from build123d import *

# Parameters (mm, degrees)
SKETCH2_W           = 38.1
SKETCH2_H           = 63.5
SKETCH2_R           = 2.1844
SKETCH2_W_2         = 19.939
SKETCH2_H_2         = 40.005
BOSS_EXTRUDE1_DEPTH = 3.175
SKETCH4_W           = 71.079825169
SKETCH4_H           = 63.5
SKETCH4_R           = 14.2875
SKETCH4_R_2         = 2.54
BOSS_EXTRUDE3_DEPTH = 3.175


with BuildPart() as part:
    # Sketch2 → Boss-Extrude1 (new body)
    with BuildSketch(Plane(origin=(0, 0, 0), x_dir=(1, 0, 0), z_dir=(0, 1, 0))):
        with Locations((0, -10.3505)):
            Rectangle(SKETCH2_W, SKETCH2_H)
        with Locations(Location((5.08, 13.462, 0), (0, 0, 270))):
            Circle(SKETCH2_R, mode=Mode.SUBTRACT)
        with Locations(Location((-5.08, 13.462, 0), (0, 0, 270))):
            Circle(SKETCH2_R, mode=Mode.SUBTRACT)
        with Locations(Location((-5.08, -34.163, 0), (0, 0, 270))):
            Circle(SKETCH2_R, mode=Mode.SUBTRACT)
        with Locations(Location((5.08, -34.163, 0), (0, 0, 270))):
            Circle(SKETCH2_R, mode=Mode.SUBTRACT)
        with Locations((0, -10.3505)):
            Rectangle(SKETCH2_W_2, SKETCH2_H_2, mode=Mode.SUBTRACT)
    extrude(amount=BOSS_EXTRUDE1_DEPTH)

    # Sketch4 → Boss-Extrude3 (add, through all)
    with BuildSketch(Plane(origin=(0, 3.175, 0), x_dir=(1, 0, 0), z_dir=(0, 1, 0))):
        with Locations((-54.589912584, -10.3505)):
            Rectangle(SKETCH4_W, SKETCH4_H)
        with Locations(Location((-54.589912585, -10.3505, 0), (0, 0, 270))):
            Circle(SKETCH4_R, mode=Mode.SUBTRACT)
        with Locations(Location((-83.779825169, 15.0495, 0), (0, 0, 270))):
            Circle(SKETCH4_R_2, mode=Mode.SUBTRACT)
        with Locations(Location((-25.4, 15.0495, 0), (0, 0, 270))):
            Circle(SKETCH4_R_2, mode=Mode.SUBTRACT)
        with Locations(Location((-25.4, -35.7505, 0), (0, 0, 270))):
            Circle(SKETCH4_R_2, mode=Mode.SUBTRACT)
        with Locations(Location((-83.779825169, -35.7505, 0), (0, 0, 270))):
            Circle(SKETCH4_R_2, mode=Mode.SUBTRACT)
    extrude(amount=-BOSS_EXTRUDE3_DEPTH)


solid = part.part
The listing builds one solid part. Answer for the finished solid, in the listing's coordinates (mm). A direction names the side the tool comes from. Round coordinates to 2 decimals unless told otherwise and drop trailing zeros. Order: outer loops, then holes, each group sorted by start corner. A loop starts at its lowest first (then second) coordinate and runs counter-clockwise, first axis right, second up. Notation, with made-up numbers: (2.5, -11) -> (47.5, -11) arc R19 cw to (47.5, 8) -> close; hole circle Ø1 at (-33, -11.5). An arc over 180 degrees is marked (long way). Put each result on its own line as item: value.
Q1. Section D-D, the plane y = 1.6 is taken. Count the separate pieces of the cut face and the enclosed holes in it, and give its area (3 significant figures).
Results list:
separate pieces: 1
enclosed holes: 10
area: 5,350 mm^2
Q2. Consider line 1 along X through (y, z) = (0.2, 10); line 2 along Z through (x, y) = (5, 1.7); line 3 along X through (y, z) = (2.05, 3). Determine where each line is inside the solid, lowest interval first.
Results list:
line 1: -90.13 to -68.87, -40.31 to -9.97, 9.97 to 19.05
line 2: -21.4 to -15.64, -11.28 to -9.65, 30.35 to 31.98, 36.35 to 42.1
line 3: -90.13 to -66.84, -42.34 to -9.97, 9.97 to 19.05
Q3. Which of the six approach directions +Z, -Z, +X, -X, +Y, -Y give full straight-line access (tool end or side, diameter ignored) to faces 5 (the flat face through (-90.13, 2, 11)), 6 (the flat face through (0, 2, -9.652))?
Results list:
face 5: +Z, -Z, -X, +Y, -Y
face 6: +Y, -Y
Q4. Section C-C, the plane x = 5.08 is taken. Write down the section's boundary in (y, z) (1 decimal), and give its area (3 significant figures).
Results list:
outline: (0, -21.4) -> (3.2, -21.4) -> (3.2, -15.6) -> (0, -15.6) -> close; (0, -11.3) -> (3.2, -11.3) -> (3.2, -9.7) -> (0, -9.7) -> close; (0, 30.4) -> (3.2, 30.4) -> (3.2, 32) -> (0, 32) -> close; (0, 36.3) -> (3.2, 36.3) -> (3.2, 42.1) -> (0, 42.1) -> close
area: 46.9 mm^2
Q5. Section A-A, the plane x = -25.4 is taken. Write down the section's boundary in (y, z) (1 decimal).
Results list:
outline: (0, -21.4) -> (3.2, -21.4) -> (3.2, -17.6) -> (0, -17.6) -> close; (0, -12.5) -> (3.2, -12.5) -> (3.2, 33.2) -> (0, 33.2) -> close; (0, 38.3) -> (3.2, 38.3) -> (3.2, 42.1) -> (0, 42.1) -> close
Q6. Determine the mould class of faces 1 (the flat face through (9.97, 2, 11)), 2 (the flat face through (-36, 0, 10)), 3 (the flat face through (19.05, 2, 11)), 4 (the flat face through (0, 2, 30.353)) for opening direction X: pulls with the +X half, pulls with the -X half, needs draft (parallel to the pull), parting line crosses it, or undercut.
Results list:
face 1: undercut
face 2: needs draft
face 3: pulls with the +X half
face 4: undercut
